from build123d import *

# Parameters (mm, degrees)
BOSS_EXTRUDE1_DEPTH = 10
CHAMFER1_SIZE       = 2
FILLET1_R           = 0.7
FILLET2_R           = 0.3


with BuildPart() as part:
    # Sketch1 → Boss-Extrude1 (new body)
    with BuildSketch(Plane(origin=(0, 0, 0), x_dir=(1, 0, 0), z_dir=(0, 1, 0))):
        Polygon((-1.7, -14.845158122), (-1.7, -7.845158122), (-6.7, -7.845158122), (-6.7, -3.845158122), (7.3, -3.845158122), (7.3, -7.845158122), (2.3, -7.845158122), (2.3, -14.845158122), (3.8, -14.845158122), (5.3, -11.845158122), (3.8, -11.845158122), (3.8, -9.345158122), (8.8, -9.345158122), (8.8, -2.345158122), (-8.2, -2.345158122), (-8.2, -9.345158122), (-3.2, -9.345158122), (-3.2, -11.845158122), (-4.7, -11.845158122), (-3.2, -14.845158122), align=None)
    extrude(amount=BOSS_EXTRUDE1_DEPTH)

    # Chamfer1
    chamfer1_edges = [part.edges().sort_by_distance(p)[0] for p in [
        (-8.2, 5, 2.345158122),
        (8.8, 5, 2.345158122),
        (7.3, 5, 3.845158122),
        (-6.7, 5, 3.845158122),
    ]]
    chamfer(chamfer1_edges, length=CHAMFER1_SIZE)

    # Fillet1
    fillet1_edges = [part.edges().sort_by_distance(p)[0] for p in [
        (-1.7, 5, 14.845158122),
        (-3.2, 5, 14.845158122),
        (-8.2, 5, 9.345158122),
        (8.8, 5, 9.345158122),
        (3.8, 5, 14.845158122),
        (2.3, 5, 14.845158122),
        (2.3, 5, 7.845158122),
        (-1.7, 5, 7.845158122),
        (-8.2, 5, 4.345158122),
        (6.8, 5, 2.345158122),
        (-6.2, 5, 2.345158122),
        (8.8, 5, 4.345158122),
    ]]
    fillet(fillet1_edges, radius=FILLET1_R)

    # Fillet2
    fillet2_edges = [part.edges().sort_by_distance(p)[0] for p in [
        (-4.7, 5, 11.845158122),
        (5.3, 5, 11.845158122),
    ]]
    fillet(fillet2_edges, radius=FILLET2_R)


solid = part.part
Here's how the part is built. I have some questions about the finished solid (model axes, mm). A direction names the side the tool comes from. Coordinates: 2 decimals unless noted, no trailing zeros. Write each loop counter-clockwise with the first axis right and the second up, starting at its lowest first coordinate (ties: lowest second). Pieces come first, ordered by that corner, then holes. Notation, with made-up numbers: (47.5, -30) - (60.5, -30) arc R22 ccw to (60.5, 6) - close; hole circle Ø3 at (-8, 73). An arc over 180 degrees is marked (long way). Use one line per item in the form item = value.
1) Suppose I cut it at B-B, the plane x = 2.75. Write out the boundary of the cut face in (y, z), plus the area to 3 significant figures.
Solved:
outline = (0, 2.35) - (10, 2.35) - (10, 3.85) - (0, 3.85) - close; (0, 7.89) - (10, 7.89) - (10, 14.8) - (0, 14.8) - close
area = 84.1 mm2
2) On a 3-axis mill with a long thin cutter (end or side, diameter ignored), from which of +Z, -Z, +X, -X, +Y, -Y can I reach the whole of each face in a straight line? I mean faces 4 (the flat face through (3.8, 5, 11)), 5 (the flat face through (-3.2, 5, 11)), 6 (the flat face through (6.314, 4.93, 4.859)), 7 (the flat face through (2.3, 5, 11)). Say none if no direction works.
Solved:
face_4 = +X, +Y, -Y
face_5 = -X, +Y, -Y
face_6 = +Y, -Y
face_7 = +Z, +Y, -Y
3) I'm going to push flat-ended pins straight in: P1, Ø3, axis at y = 3.5, z = 11, coming from the +X side; P2, Ø0.8, axis at y = 4, z = 10.5, coming from the +X side; P3, Ø6, axis at y = 4, z = 12, coming from the -X side. Where does each tip first touch, or does it pass through?
Solved:
P1 = 5.11
P2 = 3.8
P3 = -8.1
4) Thinking about a two-plate mould opening in X: for faces 1 (the flat face through (3, 0, 8)), 2 (the flat face through (0, 5, 3.845)), 3 (the flat face through (-3.946, 4.93, 13.354)), which applies, released by +X, released by -X, zero draft, split by the parting line, or undercut?
Solved:
face_1 = zero draft
face_2 = undercut
face_3 = released by -X
5) I need wall thicknesses on line 1 (Z direction, x = -2.5, y = 3.25); line 2 (X direction, y = 1.25, z = 10.5); line 3 (X direction, y = 0.75, z = 7). Which ranges of each line are inside material? Lowest first, please.
Solved:
line_1 = 2.35 to 3.85, 7.85 to 14.85
line_2 = -3.2 to -1.7, 2.3 to 3.8
line_3 = -8.2 to -6.7, 7.3 to 8.8
6) Suppose I cut it at A-A, the plane z = 7.25. Write out the boundary of the cut face in (x, y).
Solved:
outline = (-8.2, 0) - (-6.7, 0) - (-6.7, 10) - (-8.2, 10) - close; (7.3, 0) - (8.8, 0) - (8.8, 10) - (7.3, 10) - close
